Input: part model. Units: mm. Frame: model coordinates. A direction names the side the tool comes from. Give positions to 0.01 mm unless a question says otherwise; leave off trailing zeros. Order: outer loops, then holes, each group sorted by start corner. A loop starts at its lowest first (then second) coordinate and runs counter-clockwise, first axis right, second up. Notation, with made-up numbers: (-4, -34.5) - (54, -34.5) arc R25 cw to (54, -2.5) - close; hole circle Ø3 at (54.5, -28). An arc over 180 degrees is marked (long way). Answer in a Markdown table with one row per item. Add a question column.
from build123d import *

# Parameters (mm, degrees)
SKETCH1_W           = 66.5
SKETCH1_H           = 27
SKETCH1_R           = 1.5
BOSS_EXTRUDE1_DEPTH = 0.5
SKETCH2_W           = 5
SKETCH2_H           = 2.5
SKETCH2_W_2         = 4.4
SKETCH2_H_2         = 1.9
BOSS_EXTRUDE2_DEPTH = 5
SKETCH4_W           = 4
SKETCH4_H           = 7
SKETCH4_W_2         = 3.2
SKETCH4_H_2         = 6.2
BOSS_EXTRUDE3_DEPTH = 5


with BuildPart() as part:
    # Sketch1 → Boss-Extrude1 (new body)
    with BuildSketch(Plane(origin=(0, 0, 0), x_dir=(1, 0, 0), z_dir=(0, 1, 0))):
        Rectangle(SKETCH1_W, SKETCH1_H)
        with Locations(Location((-30, 9, 0), (0, 0, 270))):
            Circle(SKETCH1_R, mode=Mode.SUBTRACT)
        with Locations(Location((-30, -9, 0), (0, 0, 270))):
            Circle(SKETCH1_R, mode=Mode.SUBTRACT)
        with Locations(Location((30, 9, 0), (0, 0, 270))):
            Circle(SKETCH1_R, mode=Mode.SUBTRACT)
        with Locations(Location((30, -9, 0), (0, 0, 270))):
            Circle(SKETCH1_R, mode=Mode.SUBTRACT)
    extrude(amount=BOSS_EXTRUDE1_DEPTH)

    # Sketch2 → Boss-Extrude2 (add)
    # profile 1 of 4: a face of its own
    with BuildSketch(Plane(origin=(0, 0.5, 0), x_dir=(1, 0, 0), z_dir=(0, 1, 0))):
        with Locations((-21.228920611, 7.25)):
            Rectangle(SKETCH2_W, SKETCH2_H)
        with Locations((-21.228920611, 7.25)):
            Rectangle(SKETCH2_W_2, SKETCH2_H_2, mode=Mode.SUBTRACT)
    # profile 2 of 4: a face of its own
    with BuildSketch(Plane(origin=(0, 0.5, 0), x_dir=(1, 0, 0), z_dir=(0, 1, 0))):
        with Locations((-12.228920611, 7.25)):
            Rectangle(SKETCH2_W, SKETCH2_H)
        with Locations((-12.228920611, 7.25)):
            Rectangle(SKETCH2_W_2, SKETCH2_H_2, mode=Mode.SUBTRACT)
    # profile 3 of 4: a face of its own
    with BuildSketch(Plane(origin=(0, 0.5, 0), x_dir=(1, 0, 0), z_dir=(0, 1, 0))):
        with Locations((-12.228920611, -7.25)):
            Rectangle(SKETCH2_W, SKETCH2_H)
        with Locations((-12.228920611, -7.25)):
            Rectangle(SKETCH2_W_2, SKETCH2_H_2, mode=Mode.SUBTRACT)
    # profile 4 of 4: a face of its own
    with BuildSketch(Plane(origin=(0, 0.5, 0), x_dir=(1, 0, 0), z_dir=(0, 1, 0))):
        with Locations((-21.228920611, -7.25)):
            Rectangle(SKETCH2_W, SKETCH2_H)
        with Locations((-21.228920611, -7.25)):
            Rectangle(SKETCH2_W_2, SKETCH2_H_2, mode=Mode.SUBTRACT)
    extrude(amount=BOSS_EXTRUDE2_DEPTH)

    # Sketch4 → Boss-Extrude3 (add)
    with BuildSketch(Plane(origin=(0, 0.5, 0), x_dir=(1, 0, 0), z_dir=(0, 1, 0))):
        with Locations((-5.732400649, 0.074372007)):
            Rectangle(SKETCH4_W, SKETCH4_H)
        with Locations((-5.732400649, 0.074372007)):
            Rectangle(SKETCH4_W_2, SKETCH4_H_2, mode=Mode.SUBTRACT)
    extrude(amount=BOSS_EXTRUDE3_DEPTH)


solid = part.part
Q1. Contact query for flat-ended pins moving along their axis: P1, Ø3, axis at y = 2.5, z = 7, coming from the -X side; P2, Ø2.5, axis at x = -5.5, y = 4, coming from the -Z side; P3, Ø2, axis at x = -21.5, y = 2, coming from the -Z side. Output: stop coordinate, or through.
Q2. Section D-D, the plane x = 13.5. Return loops of the section in (y, z).
Q3. Pull-direction query (X, two-part tool) for faces 5 (the cylindrical face through (31.01, 0.25, -10.11)), 6 (the flat face through (-23.729, 3, -7)), 7 (the flat face through (0, 0, 0)); classes: +X half, -X half, draft (parallel to the pull), parting line (faces both ways), or undercut.
Q4. Section C-C, the plane z = -1.5. Return loops of the section in (x, y).
Q5. Section A-A, the plane x = 30. Return loops of the section in (y, z), then the cut area to 3 significant figures.
Q6. Access query for faces 1 (the flat face through (-6, 3, -3.574)), 2 (the flat face through (-6, 0.5, 0)), 3 (the flat face through (-18.729, 3, 7)), 4 (the flat face through (-21, 3, 8.5)). Directions: +Z, -Z, +X, -X, +Y, -Y. A direction counts if a zero-diameter tool reaches every point of the face in a straight line with its end or side. Return the directions, or none.
Q7. Line query: probe 1 along Z at (x, y) = (-19.5, 4.8); probe 2 along X at (y, z) = (2.4, 2); probe 3 along Z at (x, y) = (-14.5, 4.8). Output: solid intervals per line, ascending.
Q8. Section B-B, the plane y = 4.4. State how many separate pieces and enclosed holes the cut face has, then the cut area to 3 significant figures.
Computed:
| question | item | result |
|---|---|---|
| 1 | P1 | stops at x = -23.73 |
| 1 | P2 | stops at z = -3.57 |
| 1 | P3 | stops at z = -8.5 |
| 2 | outline | (0, -13.5) - (0.5, -13.5) - (0.5, 13.5) - (0, 13.5) - close |
| 3 | face 5 | undercut |
| 3 | face 6 | -X half |
| 3 | face 7 | draft |
| 4 | outline | (-33.25, 0) - (33.25, 0) - (33.25, 0.5) - (-3.73, 0.5) - (-3.73, 5.5) - (-4.13, 5.5) - (-4.13, 0.5) - (-7.33, 0.5) - (-7.33, 5.5) - (-7.73, 5.5) - (-7.73, 0.5) - (-33.25, 0.5) - close |
| 5 | outline | (0, -13.5) - (0.5, -13.5) - (0.5, -10.5) - (0, -10.5) - close; (0, -7.5) - (0.5, -7.5) - (0.5, 7.5) - (0, 7.5) - close; (0, 10.5) - (0.5, 10.5) - (0.5, 13.5) - (0, 13.5) - close |
| 5 | area | 10.5 mm^2 |
| 6 | face 1 | -Z, +X, -X, +Y |
| 6 | face 2 | +Y |
| 6 | face 3 | +Z, -Z, +Y |
| 6 | face 4 | +Z, +X, -X, +Y |
| 7 | probe 1 | z = -8.5 to -8.2, -6.3 to -6, 6 to 6.3, 8.2 to 8.5 |
| 7 | probe 2 | x = -7.73 to -7.33, -4.13 to -3.73 |
| 7 | probe 3 | z = -8.5 to -6, 6 to 8.5 |
| 8 | separate pieces | 5 |
| 8 | enclosed holes | 5 |
| 8 | area | 24.7 mm^2 |
